from build123d import *

# Parameters (mm, degrees)
SKETCH1_W           = 52
SKETCH1_H           = 220
BOSS_EXTRUDE1_DEPTH = 8
SKETCH2_W           = 7
SKETCH2_H           = 220
BOSS_EXTRUDE2_DEPTH = 80
SKETCH3_W           = 45
SKETCH3_H           = 7
BOSS_EXTRUDE3_DEPTH = 80
SKETCH4_W           = 45
SKETCH4_H           = 7
BOSS_EXTRUDE4_DEPTH = 80
SKETCH8_W           = 200
SKETCH8_H           = 80
CUT_EXTRUDE3_DEPTH  = 10
SKETCH10_R          = 2.2
CUT_EXTRUDE5_DEPTH  = 8
SKETCH11_W          = 7
SKETCH11_H          = 206
SKETCH11_H_2        = 200
BOSS_EXTRUDE6_DEPTH = 3
SKETCH12_W          = 7
SKETCH12_H          = 3
BOSS_EXTRUDE7_DEPTH = 77
SKETCH13_R          = 4
CUT_EXTRUDE6_DEPTH  = 2


with BuildPart() as part:
    # Sketch1 → Boss-Extrude1 (new body)
    with BuildSketch(Plane(origin=(0, 0, 0), x_dir=(1, 0, 0), z_dir=(0, 1, 0))):
        with Locations((33.761174554, -57.057839406)):
            Rectangle(SKETCH1_W, SKETCH1_H)
    extrude(amount=BOSS_EXTRUDE1_DEPTH)

    # Sketch2 → Boss-Extrude2 (add)
    with BuildSketch(Plane(origin=(0, 8, 0), x_dir=(1, 0, 0), z_dir=(0, 1, 0))):
        with Locations((11.261174554, -57.057839406)):
            Rectangle(SKETCH2_W, SKETCH2_H)
    extrude(amount=BOSS_EXTRUDE2_DEPTH)

    # Sketch3 → Boss-Extrude3 (add)
    with BuildSketch(Plane(origin=(0, 8, 0), x_dir=(1, 0, 0), z_dir=(0, 1, 0))):
        with Locations((37.261174554, -163.557839406)):
            Rectangle(SKETCH3_W, SKETCH3_H)
    extrude(amount=BOSS_EXTRUDE3_DEPTH)

    # Sketch4 → Boss-Extrude4 (add)
    with BuildSketch(Plane(origin=(0, 8, 0), x_dir=(1, 0, 0), z_dir=(0, 1, 0))):
        with Locations((37.261174554, 49.442160594)):
            Rectangle(SKETCH4_W, SKETCH4_H)
    extrude(amount=BOSS_EXTRUDE4_DEPTH)

    # Sketch8 → Cut-Extrude3 (cut)
    with BuildSketch(Plane.ZY.offset(-7.761174554)):
        with Locations((57.057839406, 48)):
            Rectangle(SKETCH8_W, SKETCH8_H)
    extrude(amount=-CUT_EXTRUDE3_DEPTH, mode=Mode.SUBTRACT)

    # Sketch10 → Cut-Extrude5 (cut)
    with BuildSketch(Plane.XZ):
        with Locations(Location((24.761174554, 154.057839406, 0), (0, 0, 270))):
            Circle(SKETCH10_R)
        with Locations(Location((42.761174554, 154.057839406, 0), (0, 0, 270))):
            Circle(SKETCH10_R)
        with Locations(Location((42.761174554, 130.057839406, 0), (0, 0, 270))):
            Circle(SKETCH10_R)
        with Locations(Location((24.761174554, 130.057839406, 0), (0, 0, 270))):
            Circle(SKETCH10_R)
        with Locations(Location((24.761174554, -15.942160594, 0), (0, 0, 270))):
            Circle(SKETCH10_R)
        with Locations(Location((42.761174554, -15.942160594, 0), (0, 0, 270))):
            Circle(SKETCH10_R)
        with Locations(Location((42.761174554, -39.942160594, 0), (0, 0, 270))):
            Circle(SKETCH10_R)
        with Locations(Location((24.761174554, -39.942160594, 0), (0, 0, 270))):
            Circle(SKETCH10_R)
    extrude(amount=-CUT_EXTRUDE5_DEPTH, mode=Mode.SUBTRACT)

    # Sketch11 → Boss-Extrude6 (add)
    with BuildSketch(Plane(origin=(0, 8, 0), x_dir=(1, 0, 0), z_dir=(0, 1, 0))):
        with Locations((56.261174554, -57.057839406)):
            Rectangle(SKETCH11_W, SKETCH11_H)
        with Locations((11.261174554, -57.057839406)):
            Rectangle(SKETCH11_W, SKETCH11_H_2)
    extrude(amount=BOSS_EXTRUDE6_DEPTH)

    # Sketch12 → Boss-Extrude7 (add)
    with BuildSketch(Plane(origin=(0, 88, 0), x_dir=(1, 0, 0), z_dir=(0, 1, 0))):
        with Locations((56.261174554, 44.442160594)):
            Rectangle(SKETCH12_W, SKETCH12_H)
        with Locations((56.261174554, -158.557839406)):
            Rectangle(SKETCH12_W, SKETCH12_H)
    extrude(amount=-BOSS_EXTRUDE7_DEPTH)

    # Sketch13 → Cut-Extrude6 (cut)
    with BuildSketch(Plane(origin=(0, 8, 0), x_dir=(1, 0, 0), z_dir=(0, 1, 0))):
        with Locations(Location((42.761174554, -154.057839406, 0), (0, 0, 270))):
            Circle(SKETCH13_R)
        with Locations(Location((24.761174554, -154.057839406, 0), (0, 0, 270))):
            Circle(SKETCH13_R)
        with Locations(Location((24.761174554, -130.057839406, 0), (0, 0, 270))):
            Circle(SKETCH13_R)
        with Locations(Location((42.761174554, -130.057839406, 0), (0, 0, 270))):
            Circle(SKETCH13_R)
        with Locations(Location((42.761174554, 15.942160594, 0), (0, 0, 270))):
            Circle(SKETCH13_R)
        with Locations(Location((24.761174554, 15.942160594, 0), (0, 0, 270))):
            Circle(SKETCH13_R)
        with Locations(Location((24.761174554, 39.942160594, 0), (0, 0, 270))):
            Circle(SKETCH13_R)
        with Locations(Location((42.761174554, 39.942160594, 0), (0, 0, 270))):
            Circle(SKETCH13_R)
    extrude(amount=-CUT_EXTRUDE6_DEPTH, mode=Mode.SUBTRACT)


solid = part.part
The model under review builds one solid part; all positions refer to its coordinate system, in mm. A direction names the side the tool comes from. Give positions to 0.01 mm unless a question says otherwise; leave off trailing zeros. Loops run counter-clockwise (first coordinate to the right, second up) from the corner with the lowest first, then second, coordinate; pieces in that order, holes last. Notation, with made-up numbers: (15.25, 66) -> (51.25, 66) arc R27 cw to (51.25, 101) -> close; hole circle Ø4 at (-3.5, 21.25). An arc over 180 degrees is marked (long way). Put each result on its own line as item: value. Start each with the question number.
1. We need section B-B on z = -22. State the section outline as (x, y) points, then the cut area to 3 significant figures.
2. Clearance check with flat-ended pins moving along their axes: P1, Ø3.5, axis at x = 9.5, z = 12, coming from the +Y side; P2, Ø6.5, axis at x = 23.5, z = 130.5, coming from the +Y side; P3, Ø3.5, axis at x = 24.76, z = -39.94, coming from the +Y side; P4, Ø2.5, axis at x = 44.5, z = 131, coming from the +Y side. State where each tip first meets the part, or that it passes through.
3. We need section A-A on y = 29. State the section outline as (x, z) points, then the cut area to 3 significant figures.
4. For faces 1 (the face through (11, 49, 157.058)), 2 (the face through (40.33, 7.01, 150.88)), 3 (the face through (33, 43, -52.942)), list the 3-axis set-ups (+Z, -Z, +X, -X, +Y, -Y) from which the entire face can be reached by the end or side of a thin tool; tool diameter is ignored.
5. Mouldability with a two-part tool opening along X and no side actions: class faces 4 (the face through (33, 88, 163)), 5 (the face through (59.761, 5, 58)), 6 (the face through (43.42, 2.96, 151.96)) as released by +X, released by -X, zero draft, split by the parting line, or undercut.
6. Wall thickness on probe 1 along Z at (x, y) = (27, 70.5); probe 2 along Y at (x, z) = (49.5, -5); probe 3 along Z at (x, y) = (10.5, 84): over which ranges is each line inside the solid? List them lowest first.
7. We need section C-C on x = 17.5. State the section outline as (y, z) points, then the cut area to 3 significant figures.
Determined:
1. outline: (7.76, 0) -> (59.76, 0) -> (59.76, 11) -> (52.76, 11) -> (52.76, 8) -> (14.76, 8) -> (14.76, 11) -> (7.76, 11) -> close
1. area: 458 mm^2
2. P1: y = 11
2. P2: y = 8
2. P3: through
2. P4: y = 6
3. outline: (7.76, -52.94) -> (59.76, -52.94) -> (59.76, -42.94) -> (52.76, -42.94) -> (52.76, -45.94) -> (14.76, -45.94) -> (14.76, -42.94) -> (7.76, -42.94) -> close; (7.76, 157.06) -> (14.76, 157.06) -> (14.76, 160.06) -> (52.76, 160.06) -> (52.76, 157.06) -> (59.76, 157.06) -> (59.76, 167.06) -> (7.76, 167.06) -> close
3. area: 812 mm^2
4. face 1: +X, -X, +Y
4. face 2: +Y
4. face 3: -Z, +X, -X, +Y, -Y
5. face 4: zero draft
5. face 5: released by +X
5. face 6: undercut
6. probe 1: -52.94 to -45.94, 160.06 to 167.06
6. probe 2: 0 to 8
6. probe 3: -52.94 to -42.94, 157.06 to 167.06
7. outline: (0, -52.94) -> (88, -52.94) -> (88, -45.94) -> (8, -45.94) -> (8, 160.06) -> (88, 160.06) -> (88, 167.06) -> (0, 167.06) -> close
7. area: 2,880 mm^2
